The listing builds one solid part. Answer for the finished solid, in the listing's coordinates (mm). Give positions to 0.01 mm unless a question says otherwise; leave off trailing zeros. Loops run counter-clockwise (first coordinate to the right, second up) from the corner with the lowest first, then second, coordinate; pieces in that order, holes last. Notation, with made-up numbers: (75, 59) - (127, 59) arc R6 cw to (127, 68) - close; hole circle Ø7 at (16, -2). An arc over 180 degrees is marked (long way). Write item = value, one per line. Start each with the question number.
1) Consider probe 1 along Y at (x, z) = (0, -0.75); probe 2 along X at (y, z) = (-14, -3.25); probe 3 along X at (y, z) = (71.5, 2.5). Determine where each line is inside the solid, lowest interval first.
2) Flat-ended cylindrical pins translate along their axes: P1, Ø5, axis at y = -92, z = 2.5, coming from the +X side; P2, Ø6, axis at x = 86, z = 2, coming from the -Y side; P3, Ø2, axis at x = 4, z = -1, coming from the -Y side. Find the tip coordinate at first contact, or state that the pin passes through.
3) The part is cut by section B-B on x = -38. Write down the section's boundary in (y, z), plus the area to 3 significant figures.
4) The part is cut by section D-D on y = 57.5. Write down the section's boundary in (x, z), plus the area to 3 significant figures.
5) The part is cut by section A-A on y = -19.5. Write down the section's boundary in (x, z).
6) The part is cut by section C-C on z = 3.25. Write down the section's boundary in (x, y), plus the area to 3 significant figures.
from build123d import *

# Parameters (mm, degrees)
SKETCH1_R          = 125
SKETCH1_R_2        = 105
BODY_DEPTH         = 5
SKETCH2_R          = 4
CUT_EXTRUDE1_DEPTH = 11
HOLES_COUNT        = 6


with BuildPart() as part:
    # Sketch1 → Body (new body, symmetric)
    with BuildSketch(Plane.XY):
        Circle(SKETCH1_R)
        Circle(SKETCH1_R_2, mode=Mode.SUBTRACT)
    extrude(amount=BODY_DEPTH, both=True)

    # Sketch2 → Cut-Extrude1 (cut, through all)
    with BuildSketch(Plane.XY.offset(5)):
        with Locations((0, 115)):
            Circle(SKETCH2_R)
    cut_extrude1 = extrude(amount=-CUT_EXTRUDE1_DEPTH, mode=Mode.SUBTRACT)

    # Holes: Cut-Extrude1 ×6 about axis
    holes_axis = Axis((0, 0, 0), (0, 0, 1))
    for i in range(1, HOLES_COUNT):
        add(cut_extrude1.rotate(holes_axis, i * 360 / HOLES_COUNT), mode=Mode.SUBTRACT)


solid = part.part
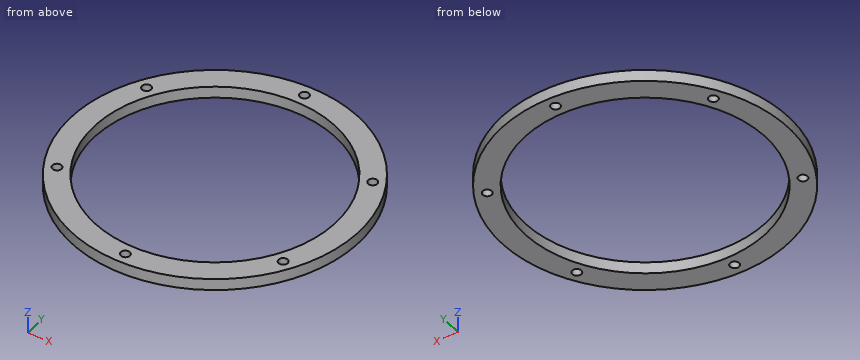
Answer below:
q1.probe_1 = -125 to -119, -111 to -105, 105 to 111, 119 to 125
q1.probe_2 = -124.21 to -104.06, 104.06 to 124.21
q1.probe_3 = -102.53 to -76.89, 76.89 to 102.53
q2.P1 = 87.26
q2.P2 = -93.47
q2.P3 = -124.96
q3.outline = (-119.08, -5) - (-97.88, -5) - (-97.88, 5) - (-119.08, 5) - close; (97.88, -5) - (119.08, -5) - (119.08, 5) - (97.88, 5) - close
q3.area = 424 mm2
q4.outline = (-110.99, -5) - (-103.59, -5) - (-103.59, 5) - (-110.99, 5) - close; (-95.59, -5) - (-87.86, -5) - (-87.86, 5) - (-95.59, 5) - close; (87.86, -5) - (95.59, -5) - (95.59, 5) - (87.86, 5) - close; (103.59, -5) - (110.99, -5) - (110.99, 5) - (103.59, 5) - close
q4.area = 303 mm2
q5.outline = (-123.47, -5) - (-103.17, -5) - (-103.17, 5) - (-123.47, 5) - close; (103.17, -5) - (123.47, -5) - (123.47, 5) - (103.17, 5) - close
q6.outline = circle Ø250 at (0, 0); hole circle Ø210 at (0, 0); hole circle Ø8 at (-99.59, -57.5); hole circle Ø8 at (-99.59, 57.5); hole circle Ø8 at (0, -115); hole circle Ø8 at (0, 115); hole circle Ø8 at (99.59, -57.5); hole circle Ø8 at (99.59, 57.5)
q6.area = 14,100 mm2
